Check sheet for the modelled part. Datum: model origin and axes. Units: mm. A direction names the side the tool comes from. Give positions to 0.01 mm unless a question says otherwise; leave off trailing zeros. Loops run counter-clockwise (first coordinate to the right, second up) from the corner with the lowest first, then second, coordinate; pieces in that order, holes last. Notation, with made-up numbers: (10, -32.75) -> (66, -32.75) arc R18 cw to (66, 0.25) -> close; hole circle Ø10 at (51.25, -23). An arc over 180 degrees is marked (long way). Write each question's results on one line, items separated by ' | '. Start each with the question number.
Item 1: Scan lines: line 1 along X through (y, z) = (6.75, -7); line 2 along Z through (x, y) = (-24, 5); line 3 along Y through (x, z) = (-19.5, -0.5). Record each from-to range of solid material in increasing order.
Item 2: Access from +Z, -Z, +X, -X, +Y, -Y to the whole of each face (thin tool, end or side, straight path). Record for faces 1 (the face through (25.5, 12.8, -0.2)), 2 (the face through (0, 9, -18)), 3 (the face through (-19, 12, 15.5)), 4 (the face through (18.94, 11.23, 16.9)), 5 (the face through (-18.94, 11.9, 17.64)).
Item 3: Mould release check, pull along Y, two halves, no side actions. Record for faces 6 (the face through (18.94, 11.2, -16.93)), 7 (the face through (0, 9, 18)), 8 (the face through (19, 12, 15.5)): pulls with the +Y half, pulls with the -Y half, needs draft (parallel to the pull), parting line crosses it, or undercut.
Item 4: Cross-section at A-A on y = 5.5. Enter the section's corners in (x, z).
Item 5: Cross-section at C-C on x = 10. Enter the section's corners in (y, z), then the cut area to 3 significant figures.
Item 6: Gauge pin test, flat ends, axial feed: pin 1 Ø2 at (x, z) = (7, -5.5) entering from +Y; pin 2 Ø0.8 at (x, y) = (19, 12.5) entering from +Z; pin 3 Ø1.1 at (x, y) = (19, 12.5) entering from -Z. Record the tip position at first contact, or that the pin passes through.
Item 7: Cross-section at D-D on x = 18. Enter the section's corners in (y, z), then the cut area to 3 significant figures.
Item 8: Cross-section at B-B on z = -5. Enter the section's corners in (x, y), then the cut area to 3 significant figures.
from build123d import *

# Parameters (mm, degrees)
SKETCH1_W               = 52
SKETCH1_H               = 37
BOSS_EXTRUDE1_DEPTH     = 12.8
FILLET1_R               = 3
SHELL2_START            = -25
SHELL2_DEPTH            = 50
CUT_EXTRUDE1_DEPTH      = 47.998297842
CUT_EXTRUDE1_DEPTH_BACK = 47.998297842


# Read off the part's stored shape, not the designer's step: Shell2
with BuildPart() as part:
    # Sketch1 → Boss-Extrude1 (new body)
    with BuildSketch(Plane(origin=(0, 0, 0), x_dir=(1, 0, 0), z_dir=(0, 1, 0))):
        Rectangle(SKETCH1_W, SKETCH1_H)
    extrude(amount=BOSS_EXTRUDE1_DEPTH)

    # Fillet1
    fillet1_edges = [part.edges().sort_by_distance(p)[0] for p in [
        (0, 12.8, -18.5),
        (0, 12.8, 18.5),
    ]]
    fillet(fillet1_edges, radius=FILLET1_R)

    # Shell2 outline → Shell2 (cut)
    with BuildSketch(Plane.YZ.offset(SHELL2_START)):
        with BuildLine():
            Line((12.8, 15.5), (11.8, 15.5))
            ThreePointArc((11.8, 15.5), (11.214213562, 16.914213562), (9.8, 17.5))
            Line((9.8, 17.5), (1, 17.5))
            Line((1, 17.5), (1, -17.5))
            Line((1, -17.5), (9.8, -17.5))
            ThreePointArc((9.8, -17.5), (11.214213562, -16.914213562), (11.8, -15.5))
            Line((11.8, -15.5), (12.8, -15.5))
            Line((12.8, -15.5), (12.8, 15.5))
        make_face()
    extrude(amount=SHELL2_DEPTH, mode=Mode.SUBTRACT)

    # Sketch2 → Cut-Extrude1 (cut, two sides: drawn at the far end of the back side and taken through both)
    with BuildSketch(Plane.XY.offset(18.5).offset(-CUT_EXTRUDE1_DEPTH_BACK)):
        with BuildLine():
            Line((-25, 9), (-25, 12.8))
            Line((-25, 12.8), (-22, 12.8))
            add(Edge.make_bspline(
                [(-25, 9), (-24.337551865, 9.035956423), (-22.850759104, 9.461520311), (-23.745938666, 12.539955656), (-22, 12.8)],
                knots=[0, 0, 0, 0, 0.249396221, 1, 1, 1, 1], degree=3))
        make_face()
        with BuildLine():
            Line((-16, 12.8), (16, 12.8))
            add(Edge.make_bspline(
                [(13, 9), (13.662448135, 9.035956423), (15.149240896, 9.461520311), (14.254061334, 12.539955656), (16, 12.8)],
                knots=[0, 0, 0, 0, 0.249396221, 1, 1, 1, 1], degree=3))
            Line((13, 9), (-13, 9))
            add(Edge.make_bspline(
                [(-13, 9), (-13.662448135, 9.035956423), (-15.149240896, 9.461520311), (-14.254061334, 12.539955656), (-16, 12.8)],
                knots=[0, 0, 0, 0, 0.249396221, 1, 1, 1, 1], degree=3))
        make_face()
        with BuildLine():
            Line((25, 9), (25, 12.8))
            Line((25, 12.8), (22, 12.8))
            add(Edge.make_bspline(
                [(25, 9), (24.337551865, 9.035956423), (22.850759104, 9.461520311), (23.745938666, 12.539955656), (22, 12.8)],
                knots=[0, 0, 0, 0, 0.249396221, 1, 1, 1, 1], degree=3))
        make_face()
    extrude(amount=CUT_EXTRUDE1_DEPTH + CUT_EXTRUDE1_DEPTH_BACK, mode=Mode.SUBTRACT)


solid = part.part
Answer sheet:
1) line 1: x = -26 to -25, 25 to 26 | line 2: z = -18.5 to -17.5, 17.5 to 18.5 | line 3: y = 0 to 1
2) face 1: +Z, -Z, +X, -X, +Y | face 2: +Z, -Z, +Y | face 3: +Y | face 4: none | face 5: +Z, +X, -X, +Y
3) face 6: undercut | face 7: pulls with the +Y half | face 8: needs draft
4) outline: (-26, -18.5) -> (26, -18.5) -> (26, 18.5) -> (-26, 18.5) -> close; hole (-25, -17.5) -> (25, -17.5) -> (25, 17.5) -> (-25, 17.5) -> close
5) outline: (0, -18.5) -> (9, -18.5) -> (9, -17.5) -> (1, -17.5) -> (1, 17.5) -> (9, 17.5) -> (9, 18.5) -> (0, 18.5) -> close | area: 53.0 mm²
6) pin 1: stops at y = 1 | pin 2: stops at z = 17.43 | pin 3: stops at z = -17.59
7) outline: (0, -18.5) -> (9.8, -18.5) arc R3 ccw to (12.8, -15.5) -> (11.8, -15.5) arc R2 cw to (9.8, -17.5) -> (1, -17.5) -> (1, 17.5) -> (9.8, 17.5) arc R2 cw to (11.8, 15.5) -> (12.8, 15.5) arc R3 ccw to (9.8, 18.5) -> (0, 18.5) -> close | area: 62.5 mm²
8) outline: (-26, 0) -> (26, 0) -> (26, 12.8) -> (25, 12.8) -> (25, 1) -> (-25, 1) -> (-25, 12.8) -> (-26, 12.8) -> close | area: 75.6 mm²
